Could you check a few things on this model? Use its own coordinates, in mm. Give positions to 0.01 mm unless a question says otherwise; leave off trailing zeros. Loops run counter-clockwise (first coordinate to the right, second up) from the corner with the lowest first, then second, coordinate; pieces in that order, holes last. Notation, with made-up numbers: (19, 16) - (69, 16) arc R26 cw to (69, 53) - close; hole circle Ø1 at (59, 83). An arc over 180 degrees is marked (long way). Write each question's results on one line, items separated by ' | '. Start each with the question number.
(1) For pin 1 (1 mm diameter, centred on y = -1.5, z = 55.5, fed in from -X); pin 2 (16.5 mm diameter, centred on x = 2.5, y = -13, fed in from +Z); pin 3 (5 mm diameter, centred on x = -42.5, z = 71.5, fed in from -Y), each with a flat end and sliding along its axis, tell me the tip position at first contact or that it passes through.
(2) Suppose I cut it at A-A (y = 0). Please give me the cut outline in (x, z), and give its area (3 significant figures).
(3) Suppose I cut it at D-D (z = 49.5). Please give me the cut outline in (x, y).
(4) I need wall thicknesses on line 1 (X direction, y = -43, z = 81.5); line 2 (X direction, y = -33.5, z = 32.5); line 3 (Z direction, x = 1, y = -21.5). Which ranges of each line are inside material? Lowest first, please.
(5) If we mould it in two halves opening along Y, with no side actions, what happens to faces 1 (the face through (0, 0, 12)), 2 (the face through (0, 0, 0)), 3 (the face through (-5.47, -41.64, 42.22))? For each: released by +Y, released by -Y, zero draft, split by the parting line, or undercut.
(6) Suppose I cut it at C-C (z = 65). Please give me the cut outline in (x, y).
from build123d import *


with BuildPart() as f1:
    # F0 (on Front) → F1 (revolve)
    with BuildSketch(Plane.XZ):
        with BuildLine():
            Line((0, 12), (0, 0))
            Line((0, 0), (25.467497, 0))
            ThreePointArc((25.467497, 0), (29.084074, 1.212477), (31.238978, 4.359876))
            Line((31.238978, 4.359876), (58.417735, 100))
            ThreePointArc((58.417735, 100), (57.729175, 101.235268), (56.493908, 100.546708))
            Line((56.493908, 100.546708), (32.363421, 15.63323))
            ThreePointArc((32.363421, 15.63323), (30.567667, 13.010398), (27.553853, 12))
            Line((27.553853, 12), (0, 12))
        make_face()
    revolve(axis=Axis((0, 0, 6), (0, 0, -1)))


solid = f1.part
Output values:
1) pin 1: x = -45.89 | pin 2: z = 12 | pin 3: y = -30.73
2) outline: (-58.42, 100) - (-31.24, 4.36) arc R6 ccw to (-25.47, 0) - (25.47, 0) arc R6 ccw to (31.24, 4.36) - (58.42, 100) arc R1 ccw to (56.49, 100.55) - (32.36, 15.63) arc R5 cw to (27.55, 12) - (-27.55, 12) arc R5 cw to (-32.36, 15.63) - (-56.49, 100.55) arc R1 ccw to start | area: 1,130 mm2
3) outline: circle Ø88.13 at (0, 0); hole circle Ø83.98 at (0, 0)
4) line 1: -31.26 to -27.57, 27.57 to 31.26 | line 2: -20.43 to -16.07, 16.07 to 20.43 | line 3: 0 to 12
5) face 1: undercut | face 2: zero draft | face 3: split by the parting line
6) outline: circle Ø96.94 at (0, 0); hole circle Ø92.78 at (0, 0)
